Geometry check sheet. Reference: the model listing, model coordinates, mm. A direction names the side the tool comes from. Round coordinates to 2 decimals unless told otherwise and drop trailing zeros. Write each loop counter-clockwise with the first axis right and the second up, starting at its lowest first coordinate (ties: lowest second). Pieces come first, ordered by that corner, then holes. Notation, with made-up numbers: (74.5, 56) -> (118.5, 56) arc R21 cw to (118.5, 65) -> close; hole circle Ø2 at (75.25, 47.25). An arc over 180 degrees is marked (long way). Use a Markdown table: item, result.
```python
from build123d import *

# Parameters (mm, degrees)
SKETCH1_W           = 17.805
SKETCH1_H           = 25
BOSS_EXTRUDE1_DEPTH = 3
FILLET1_R           = 2
BOSS_EXTRUDE3_DEPTH = 5
SKETCH3_R           = 1.5
CUT_EXTRUDE1_DEPTH  = 5
SKETCH7_W           = 15.61
SKETCH7_H           = 10
BOSS_EXTRUDE4_DEPTH = 30
BOSS_EXTRUDE5_DEPTH = 15.61
SKETCH9_R           = 1.5
CUT_EXTRUDE2_DEPTH  = 5
BOSS_EXTRUDE6_DEPTH = 50
FILLET2_R           = 1


with BuildPart() as part:
    # Sketch1 → Boss-Extrude1 (new body)
    with BuildSketch(Plane(origin=(0, 0, 0), x_dir=(1, 0, 0), z_dir=(0, 1, 0))):
        Polygon((9.368218391, -4.75), (-8.436781609, -4.75), (-26.241781609, -4.75), (-38.436781609, -4.75), (-38.436781609, -9.75), (21.563218391, -9.75), (21.563218391, -4.75), align=None)
        with Locations((0.465718391, 7.75)):
            Rectangle(SKETCH1_W, SKETCH1_H)
        with Locations((-17.339281609, 7.75)):
            Rectangle(SKETCH1_W, SKETCH1_H)
    extrude(amount=BOSS_EXTRUDE1_DEPTH)

    # Fillet1
    fillet1_edges = [part.edges().sort_by_distance(p)[0] for p in [
        (-8.436781609, 0, 9.75),
    ]]
    fillet(fillet1_edges, radius=FILLET1_R)

    # Sketch2 → Boss-Extrude3 (add)
    with BuildSketch(Plane(origin=(21.563218391, 0, 0), x_dir=(0, 0, -1), z_dir=(1, 0, 0))):
        with BuildLine():
            Line((-29.75, 46.301270189), (-32.25, 41.97114317))
            ThreePointArc((-32.25, 41.97114317), (-15.77885683, 25.5), (-9.75, 3))
            Line((-9.75, 3), (-4.75, 3))
            ThreePointArc((-4.75, 3), (-11.448729811, 28), (-29.75, 46.301270189))
        make_face()
    boss_extrude3 = extrude(amount=-BOSS_EXTRUDE3_DEPTH)

    # Mirror3: Boss-Extrude3 across plane
    add(boss_extrude3.mirror(Plane(origin=(-8.436781609, 0, 0), x_dir=(0, 0, 1), z_dir=(1, 0, 0))))

    # Sketch3 → Cut-Extrude1 (cut)
    with BuildSketch(Plane.XZ):
        with Locations(Location((-20.484687418, -8.75, 0), (0, 0, 270))):
            Circle(SKETCH3_R)
        with Locations(Location((-8.434877213, -16.25, 0), (0, 0, 270))):
            Circle(SKETCH3_R)
        with Locations(Location((3.614932992, -8.75, 0), (0, 0, 270))):
            Circle(SKETCH3_R)
    extrude(amount=-CUT_EXTRUDE1_DEPTH, mode=Mode.SUBTRACT)

    # Sketch7 → Boss-Extrude4 (add)
    with BuildSketch(Plane(origin=(0, 3, 0), x_dir=(1, 0, 0), z_dir=(0, 1, 0))):
        with Locations((-8.436781609, 0.25)):
            Rectangle(SKETCH7_W, SKETCH7_H)
    extrude(amount=BOSS_EXTRUDE4_DEPTH)

    # Sketch8 → Boss-Extrude5 (add)
    with BuildSketch(Plane.ZY.offset(16.241781609)):
        Polygon((-5.25, 33), (4.75, 43), (4.75, 33), align=None)
    extrude(amount=-BOSS_EXTRUDE5_DEPTH)

    # Sketch9 → Cut-Extrude2 (cut)
    with BuildSketch(Plane(origin=(0, 19.125, -19.125), x_dir=(1, 0, 0), z_dir=(0, 0.7071067811865461, -0.7071067811865489))):
        with Locations(Location((-11.436781609, -26.69328099, 0), (0, 0, 270))):
            Circle(SKETCH9_R)
        with Locations(Location((-5.436781609, -26.69328099, 0), (0, 0, 270))):
            Circle(SKETCH9_R)
    extrude(amount=-CUT_EXTRUDE2_DEPTH, mode=Mode.SUBTRACT)

    # Sketch10 → Boss-Extrude6 (add)
    with BuildSketch(Plane(origin=(-33.436781609, 0, 0), x_dir=(0, 0, -1), z_dir=(1, 0, 0))):
        with BuildLine():
            Line((-27.04523361, 38.460483912), (-23.966926234, 42.40053768))
            ThreePointArc((-23.966926234, 42.40053768), (-26.790354826, 44.451878628), (-29.75, 46.301270189))
            Line((-29.75, 46.301270189), (-32.25, 41.97114317))
            ThreePointArc((-32.25, 41.97114317), (-29.586319344, 40.306690765), (-27.04523361, 38.460483912))
        make_face()
    extrude(amount=BOSS_EXTRUDE6_DEPTH)

    # Fillet2
    fillet2_edges = [part.edges().sort_by_distance(p)[0] for p in [
        (-38.436781609, 0, 6.25),
        (21.563218391, 0, 6.25),
        (21.563218391, 2.5, 9.75),
        (-38.436781609, 2.5, 9.75),
        (-38.436781609, 1.5, 4.75),
        (21.563218391, 1.5, 4.75),
        (21.563218391, 0.585786438, 9.164213562),
        (-38.436781609, 0.585786438, 9.164213562),
        (21.563218391, 25.5, 15.77885683),
        (21.563218391, 28, 11.448729811),
        (21.563218391, 44.13620668, 31),
        (-38.436781609, 25.5, 15.77885683),
        (-38.436781609, 28, 11.448729811),
        (-38.436781609, 44.13620668, 31),
    ]]
    fillet(fillet2_edges, radius=FILLET2_R)


solid = part.part
```
(1) Section check A-A on z = -8.75. Record the cut outline in (x, y), plus the area to 3 significant figures.
A:
| item | result |
|---|---|
| outline | (-26.24, 0) -> (-21.98, 0) -> (-21.98, 3) -> (-26.24, 3) -> close; (-18.98, 0) -> (2.11, 0) -> (2.11, 3) -> (-18.98, 3) -> close; (5.11, 0) -> (9.37, 0) -> (9.37, 3) -> (5.11, 3) -> close |
| area | 88.8 mm2 |
(2) Gauge pin test, flat ends, axial feed: pin 1 Ø3.5 at (x, y) = (-29, 2) entering from -Z; pin 2 Ø11 at (y, z) = (25, -0.5) entering from -X; pin 3 Ø4.5 at (x, y) = (-10.5, 18.5) entering from -Z. Record the tip position at first contact, or that the pin passes through.
A:
| item | result |
|---|---|
| pin 1 | stops at z = 4.75 |
| pin 2 | stops at x = -16.24 |
| pin 3 | stops at z = -5.25 |
(3) Access from +Z, -Z, +X, -X, +Y, -Y to the whole of each face (thin tool, end or side, straight path). Record for faces 1 (the face through (-26.242, 1, -8)), 2 (the face through (-9, 18, -5.25)), 3 (the face through (15, 1, 4.75)), 4 (the face through (-11.42, 34.45, 3.27)).
A:
| item | result |
|---|---|
| face 1 | -Z, -X, +Y, -Y |
| face 2 | -Z, +X, -X, +Y |
| face 3 | -Z, +X, +Y, -Y |
| face 4 | none |
(4) Release check for a two-part mould opening along X. For faces 5 (the face through (-0.632, 19, 0)), 6 (the face through (16.563, 23, 13)), 7 (the face through (-9, 0, -6)) record: +X half, -X half, draft (parallel to the pull), parting line (faces both ways), or undercut.
A:
| item | result |
|---|---|
| face 5 | +X half |
| face 6 | undercut |
| face 7 | draft |
(5) Section check B-B on z = -16.25. Record the cut outline in (x, y), plus the area to 3 significant figures.
A:
| item | result |
|---|---|
| outline | (-26.24, 0) -> (-9.93, 0) -> (-9.93, 3) -> (-26.24, 3) -> close; (-6.93, 0) -> (9.37, 0) -> (9.37, 3) -> (-6.93, 3) -> close |
| area | 97.8 mm2 |
(6) Thickness scan on line 1 (X direction, y = 1.95, z = -8.75); line 2 (X direction, y = 6.5, z = 6); line 3 (Y direction, x = -23.5, z = -17). Record the ranges inside material, lowest first.
A:
| item | result |
|---|---|
| line 1 | x = -26.24 to -21.98, -18.98 to 2.11, 5.11 to 9.37 |
| line 2 | x = -38.44 to -33.44, 16.56 to 21.56 |
| line 3 | y = 0 to 3 |
(7) Section check C-C on x = -2.5. Record the cut outline in (y, z), plus the area to 3 significant figures.
A:
| item | result |
|---|---|
| outline | (0, -20.25) -> (3, -20.25) -> (3, -5.25) -> (33, -5.25) -> (43, 4.75) -> (3, 4.75) -> (3, 9.75) -> (2, 9.75) arc R2 ccw to (0, 7.75) -> close; (38.46, 27.05) -> (42.4, 23.97) arc R50 ccw to (46.3, 29.75) -> (41.97, 32.25) arc R45 cw to start |
| area | 472 mm2 |
(8) Section check D-D on y = 27. State how many separate pieces and enclosed holes the cut face has, plus the area to 3 significant figures.
A:
| item | result |
|---|---|
| separate pieces | 3 |
| enclosed holes | 0 |
| area | 213 mm2 |
